```python
from build123d import *

# Parameters (mm, degrees)
SKETCH007_W             = 18.5
SKETCH007_H             = 4
SKETCH007_W_2           = 5.2
SKETCH007_H_2           = 3.5
BODY006_PLACEMENT_ANGLE = 180
SKETCH005_W             = 40
SKETCH005_H             = 20.3
PAD006_DEPTH            = 2


with BuildPart() as audio_socket_mockup:
    # Sketch007 → Revolution001 (revolve)
    with BuildSketch(Plane.XZ):
        with Locations((9.25, 2)):
            Rectangle(SKETCH007_W, SKETCH007_H)
        with Locations((-2.6, 1.75)):
            Rectangle(SKETCH007_W_2, SKETCH007_H_2)
    revolve(axis=Axis((0, 0, 0), (1, 0, 0)))


with BuildPart() as audio_socket_mockup_1:
    # Body006 placement: moved
    add(audio_socket_mockup.part.moved(Location((18, -7.5, 11))).rotate(Axis((18, -7.5, 11), (0, 0, 1)), BODY006_PLACEMENT_ANGLE))


with BuildPart() as audio_cut:
    # Sketch005 → Pad006 (new body)
    with BuildSketch(Plane.YZ):
        with Locations((0, 10.15)):
            Rectangle(SKETCH005_W, SKETCH005_H)
    extrude(amount=PAD006_DEPTH)


with BuildPart() as audio_cut_1:
    # Body004 placement: moved
    add(audio_cut.part.moved(Location((18, 0, 0))))

    # Cut001: cut audio socket mockup
    add(audio_socket_mockup_1.part, mode=Mode.SUBTRACT)


with BuildPart() as audio_cut_2:
    # Cut001 placement: moved
    add(audio_cut_1.part.moved(Location((-1.5, 0, 0))))


solid = audio_cut_2.part
```
Verification items for the finished model (mm, model axes). Coordinates: 2 decimals unless noted, no trailing zeros. Loops run counter-clockwise (first coordinate to the right, second up) from the corner with the lowest first, then second, coordinate; pieces in that order, holes last. Notation, with made-up numbers: (45.5, 22.5) - (77.5, 22.5) arc R7 ccw to (77.5, 27.5) - close; hole circle Ø8 at (11.5, -37). An arc over 180 degrees is marked (long way). Return JSON: item names as keys, results as strings.
1. Section check C-C, the plane x = 17.45. Record the boundary of the cut face in (y, z).
Established:
{"outline": "(-20, 0) - (20, 0) - (20, 20.3) - (-20, 20.3) - close; hole circle Ø7 at (-7.5, 11)"}
2. Go/stop test with a flat-tipped pin: pin 1 (8 mm diameter, centred on y = -7.5, z = 11, fed in from -X). Record where the tip stops, or that it passes through.
Established:
{"pin 1": "stops at x = 16.5"}
3. Section check B-B, the plane y = -7.5. Record the boundary of the cut face in (x, z), then the cut area to 3 significant figures.
Established:
{"outline": "(16.5, 0) - (18.5, 0) - (18.5, 7.5) - (16.5, 7.5) - close; (16.5, 14.5) - (18.5, 14.5) - (18.5, 20.3) - (16.5, 20.3) - close", "area": "26.6 mm2"}
4. Thickness scan on L1, parallel to Y at x = 17.1, z = 11; L2, parallel to Y at x = 17.45, z = 12.5. Record the ranges inside material, lowest first.
Established:
{"L1": "y = -20 to -11, -4 to 20", "L2": "y = -20 to -10.66, -4.34 to 20"}
5. Section check A-A, the plane z = 11. Record the boundary of the cut face in (x, y), then the cut area to 3 significant figures.
Established:
{"outline": "(16.5, -20) - (18.5, -20) - (18.5, -11) - (16.5, -11) - close; (16.5, -4) - (18.5, -4) - (18.5, 20) - (16.5, 20) - close", "area": "66.0 mm2"}
6. Mould release check, pull along Z, two halves, no side actions. Record for faces 1 (the flat face through (16.5, 0, 10)), 2 (the cylindrical face through (17.486, -7.346, 7.503)), 3 (the flat face through (17, 0, 0)), 4 (the flat face through (17, 0, 20.3)): +Z half, -Z half, draft (parallel to the pull), parting line (faces both ways), or undercut.
Established:
{"face 1": "draft", "face 2": "undercut", "face 3": "-Z half", "face 4": "+Z half"}
